from build123d import *

# Parameters (mm, degrees)
BOSS_EXTRUDE1_DEPTH = 8.4
SKETCH2_R           = 1.5
SKETCH2_R_2         = 1.75
SKETCH2_W           = 60
SKETCH2_H           = 300
SKETCH2_W_2         = 9
SKETCH2_H_2         = 9
CUT_EXTRUDE1_DEPTH  = 9.4
FILLET1_R           = 20
SKETCH3_R           = 30
SKETCH3_W           = 80
SKETCH3_H           = 110
CUT_EXTRUDE2_DEPTH  = 9.4


with BuildPart() as part:
    # Sketch1 → Boss-Extrude1 (new body)
    with BuildSketch(Plane(origin=(0, 0, 0), x_dir=(1, 0, 0), z_dir=(0, 1, 0))):
        Polygon((0, 0), (-228, 0), (-228, -215), (-376.5, -347.47169509), (-376.5, -404.47169509), (-336.5, -439.9), (-291.5, -439.9), (-275.5, -405), (-210.5, -405), (-184.5, -439.9), (-18.5, -439.9), (0, -392.4), align=None)
    extrude(amount=BOSS_EXTRUDE1_DEPTH)

    # Sketch2 → Cut-Extrude1 (cut, through all)
    with BuildSketch(Plane(origin=(0, 8.4, 0), x_dir=(1, 0, 0), z_dir=(0, 1, 0))):
        with Locations((-23.1, -408.2)):
            Circle(SKETCH2_R)
        with Locations((-23.1, -382)):
            Circle(SKETCH2_R)
        with Locations((-355.4, -407.37169509)):
            Circle(SKETCH2_R)
        with Locations((-355.4, -381.77169509)):
            Circle(SKETCH2_R)
        with Locations((-163.85, -51.1)):
            Circle(SKETCH2_R_2)
        with Locations((-123.15, -51.1)):
            Circle(SKETCH2_R_2)
        with Locations((-143.5, -387)):
            Circle(SKETCH2_R_2)
        Polygon((-336.5, -340.600531429), (-228, -243.811447811), (-201.5, -243.811447811), (-201.5, -377), (-336.5, -377), align=None)
        with Locations((-143.5, -224.9)):
            Rectangle(SKETCH2_W, SKETCH2_H)
        with Locations((-23.1, -419.4)):
            Rectangle(SKETCH2_W_2, SKETCH2_H_2)
        with Locations((-23.1, -395.95)):
            Rectangle(SKETCH2_W_2, SKETCH2_H_2)
        with Locations((-355.4, -396.97169509)):
            Rectangle(SKETCH2_W_2, SKETCH2_H_2)
        with Locations((-163.85, -65.6)):
            Rectangle(SKETCH2_W_2, SKETCH2_H_2)
        with Locations((-123.15, -65.6)):
            Rectangle(SKETCH2_W_2, SKETCH2_H_2)
        with Locations((-163, -387)):
            Rectangle(SKETCH2_W_2, SKETCH2_H_2)
        with Locations((-124, -387)):
            Rectangle(SKETCH2_W_2, SKETCH2_H_2)
        with Locations((-173.4, -410)):
            Rectangle(SKETCH2_W_2, SKETCH2_H_2)
        with Locations((-113.6, -410)):
            Rectangle(SKETCH2_W_2, SKETCH2_H_2)
    extrude(amount=-CUT_EXTRUDE1_DEPTH, mode=Mode.SUBTRACT)

    # Fillet1
    fillet1_edges = [part.edges().sort_by_distance(p)[0] for p in [
        (-228, 4.2, 0),
        (0, 4.2, 0),
    ]]
    fillet(fillet1_edges, radius=FILLET1_R)

    # Sketch3 → Cut-Extrude2 (cut, through all)
    with BuildSketch(Plane(origin=(0, 8.4, 0), x_dir=(1, 0, 0), z_dir=(0, 1, 0))):
        with Locations((-53.5, -114.9)):
            Circle(SKETCH3_R)
        with Locations((-53.5, -229.9)):
            Rectangle(SKETCH3_W, SKETCH3_H)
    extrude(amount=-CUT_EXTRUDE2_DEPTH, mode=Mode.SUBTRACT)


solid = part.part
Here's how the part is built. I have some questions about the finished solid (model axes, mm). A direction names the side the tool comes from. Give positions to 0.01 mm unless a question says otherwise; leave off trailing zeros. Order: outer loops, then holes, each group sorted by start corner. A loop starts at its lowest first (then second) coordinate and runs counter-clockwise, first axis right, second up. Notation, with made-up numbers: M 10,0 L 20,0 A19 ccw 20,22 Z; hole C 22,6 d2. An arc over 180 degrees is marked long. Answer as a JSON object with one key per item and string values. Group by question number.
1) We'd pull the mould along X, two halves only. Please class faces 4 (the flat face through (-9.38, 4.14, 416.48)), 5 (the flat face through (-197.68, 4.14, 422.21)), 6 (the cylindrical face through (-221.986, 4.259, 5.703)): pulls with the +X half, pulls with the -X half, needs draft (parallel to the pull), parting line crosses it, or undercut.
2) On a 3-axis mill with a long thin cutter (end or side, diameter ignored), from which of +Z, -Z, +X, -X, +Y, -Y can I reach the whole of each face in a straight line? I mean faces 1 (the flat face through (-283.61, 4.14, 422.69)), 2 (the flat face through (-107, 8.4, 217)), 3 (the flat face through (-283.01, 4.259, 292.884)). Say none if no direction works.
3) I'm going to push flat-ended pins straight in: pin 1 Ø2 at (x, z) = (-123.15, 51.1) entering from +Y (3 decimals); pin 2 Ø2.5 at (x, y) = (-354, 3.5) entering from +Z; pin 3 Ø4 at (y, z) = (6.5, 286.5) entering from -X. Where does each tip first touch, or does it pass through?
4) Suppose I cut it at B-B, the plane x = -220. Write out the boundary of the cut face in (y, z).
5) Suppose I cut it at C-C, the plane z = 229. Write out the boundary of the cut face in (x, y).
6) Suppose I cut it at D-D, the plane y = 6.75. Count the separate pieces of the cut face and the enclosed holes in it, plus the area to 3 significant figures.
7) Please list where these lines run through material, in increasing order: L1, parallel to Z at x = -23.1, y = 2.25; L2, parallel to X at y = 5.25, z = 387; L3, parallel to X at y = 3, z = 51.1. Write a range as [from, to].
8) Suppose I cut it at A-A, the plane x = -53.5. Write out the boundary of the cut face in (y, z), plus the area to 3 significant figures.
Results found:
{
 "1": {"face 4": "pulls with the +X half", "face 5": "undercut", "face 6": "pulls with the -X half"},
 "2": {"face 1": "+Z, +Y, -Y", "face 2": "+Z, -Z, +X, -X, +Y", "face 3": "+Y, -Y"},
 "3": {"pin 1": "through", "pin 2": "z = 425.51", "pin 3": "x = -310.39"},
 "4": {"outline": "M 0,4 L 8.4,4 L 8.4,243.81 L 0,243.81 Z; M 0,377 L 8.4,377 L 8.4,405 L 0,405 Z"},
 "5": {"outline": "M -243.69,0 L -173.5,0 L -173.5,8.4 L -243.69,8.4 Z; M -113.5,0 L -93.5,0 L -93.5,8.4 L -113.5,8.4 Z; M -13.5,0 L 0,0 L 0,8.4 L -13.5,8.4 Z"},
 "6": {"separate pieces": "1", "enclosed holes": "20", "area": "76,400 mm²"},
 "7": {"L1": "[0, 174.9], [284.9, 380.5], [383.5, 391.45], [400.45, 406.7], [409.7, 414.9], [423.9, 439.9]", "L2": "[-376.5, -167.5], [-158.5, -145.25], [-141.75, -128.5], [-119.5, 0]", "L3": "[-228, -165.6], [-162.1, -124.9], [-121.4, 0]"},
 "8": {"outline": "M 0,0 L 8.4,0 L 8.4,84.9 L 0,84.9 Z; M 0,144.9 L 8.4,144.9 L 8.4,174.9 L 0,174.9 Z; M 0,284.9 L 8.4,284.9 L 8.4,439.9 L 0,439.9 Z", "area": "2,270 mm²"}
}
